from build123d import *

# Parameters (mm, degrees)
F1_DEPTH = 12.7
F3_START = 6.35
F3_DEPTH = 12.7
F4_R     = 9.525
F4_R_2   = 6.35
F5_DEPTH = 25.4


with BuildPart() as f1:
    # F0 (on Right) → F1 (new body)
    with BuildSketch(Plane.YZ):
        Polygon((-25.4, 0), (0, 0), (0, 19.05), (-6.35, 25.4), (-19.05, 25.4), (-25.4, 19.05), align=None)
    extrude(amount=-F1_DEPTH)

    # F2 (on Front) → F3 (join)
    with BuildSketch(Plane.XZ.offset(F3_START)):
        with BuildLine():
            Line((0, 19.05), (0, 0))
            Line((0, 0), (12.7, 0))
            ThreePointArc((12.7, 0), (3.175, 9.525), (12.7, 19.05))
            Line((12.7, 19.05), (0, 19.05))
        make_face()
    extrude(amount=F3_DEPTH)

    # F4 (on Front) → F5 (join)
    with BuildSketch(Plane.XZ):
        with Locations((12.7, 9.525)):
            Circle(F4_R)
        with Locations((12.7, 9.525)):
            Circle(F4_R_2, mode=Mode.SUBTRACT)
    extrude(amount=F5_DEPTH)


solid = f1.part
Check sheet for the modelled part. Datum: model origin and axes. Units: mm. A direction names the side the tool comes from. Give positions to 0.01 mm unless a question says otherwise; leave off trailing zeros. Write each loop counter-clockwise with the first axis right and the second up, starting at its lowest first coordinate (ties: lowest second). Pieces come first, ordered by that corner, then holes. Notation, with made-up numbers: (3, 61) -> (58, 61) arc R18 cw to (58, 84) -> close; hole circle Ø11 at (-24, 40.5). An arc over 180 degrees is marked (long way). One line per item, written item: value. Start each with the question number.
Item 1: Section check A-A on x = 14. Record the cut outline in (y, z).
Item 2: Section check C-C on y = -4. Record the cut outline in (x, z) (3 decimals), then the cut area to 3 significant figures.
Item 3: Draft check along Z on faces 4 (the flat face through (15, 0, 3)), 5 (the cylindrical face through (7.66, -12.52, 5.66)), 6 (the cylindrical face through (21.5, -12.52, 5.88)). Enter one of: +Z half, -Z half, draft (parallel to the pull), parting line (faces both ways), or undercut.
Item 4: Material ranges on probe 1 along X at (y, z) = (-23.5, 9.75); probe 2 along X at (y, z) = (-23.75, 8); probe 3 along Z at (x, y) = (13, -24), recorded low to high. Write a range as from..to.
Item 5: Tool access check on faces 1 (the flat face through (6, -13, 19.05)), 2 (the flat face through (0, -13, 21)), 3 (the flat face through (2, -19.05, 10)). Record the directions out of +Z, -Z, +X, -X, +Y, -Y that give a thin tool (end or side, any length) a straight path to the whole face; none if there is none.
Item 6: Section check D-D on x = -7.5. Record the cut outline in (y, z), then the cut area to 3 significant figures.
Item 7: Section check B-B on z = 13.75. Record the cut outline in (x, y).
Item 8: Gauge pin test, flat ends, axial feed: pin 1 (6 mm diameter, centred on y = -6, z = 20.5, fed in from +X); pin 2 (4 mm diameter, centred on x = 5, y = -18, fed in from +Z); pin 3 (3 mm diameter, centred on y = -19, z = 17, fed in from +X). Record the tip position at first contact, or that the pin passes through.
Results list:
1. outline: (-25.4, 0.09) -> (0, 0.09) -> (0, 3.31) -> (-25.4, 3.31) -> close; (-25.4, 15.74) -> (0, 15.74) -> (0, 18.96) -> (-25.4, 18.96) -> close
2. outline: (-12.7, 0) -> (0, 0) -> (0, 23.05) -> (-12.7, 23.05) -> close; circle Ø19.05 at (12.7, 9.525); hole circle Ø12.7 at (12.7, 9.525)
2. area: 451 mm²
3. face 4: draft
3. face 5: undercut
3. face 6: parting line
4. probe 1: -12.7..0, 3.18..6.35, 19.05..22.22
4. probe 2: -12.7..0, 3.3..6.54, 18.86..22.1
4. probe 3: 0..3.18, 15.87..19.05
5. face 1: +Z, +X, +Y, -Y
5. face 2: +Z
5. face 3: -Y
6. outline: (-25.4, 0) -> (0, 0) -> (0, 19.05) -> (-6.35, 25.4) -> (-19.05, 25.4) -> (-25.4, 19.05) -> close
6. area: 605 mm²
7. outline: (-12.7, -25.4) -> (0, -25.4) -> (0, -19.05) -> (4.16, -19.05) -> (4.16, -25.4) -> (7.96, -25.4) -> (7.96, 0) -> (4.16, 0) -> (4.16, -6.35) -> (0, -6.35) -> (0, 0) -> (-12.7, 0) -> close; (17.44, -25.4) -> (21.24, -25.4) -> (21.24, 0) -> (17.44, 0) -> close
8. pin 1: x = 17.91
8. pin 2: z = 19.05
8. pin 3: x = 20.12
